```python
from build123d import *

# Parameters (mm, degrees)
SKETCH1_R           = 14
BOSS_EXTRUDE1_DEPTH = 10
SKETCH2_R           = 2.25
CUT_EXTRUDE1_DEPTH  = 5
SKETCH3_R           = 5
CUT_EXTRUDE2_DEPTH  = 1.8
SKETCH4_W           = 10
SKETCH4_H           = 10
BOSS_EXTRUDE2_DEPTH = 8
SKETCH6_W           = 8
SKETCH6_H           = 9.912865289
BOSS_EXTRUDE3_DEPTH = 20
CUT_EXTRUDE3_DEPTH  = 30
BOSS_EXTRUDE4_DEPTH = 80
SKETCH9_W           = 60
SKETCH9_H           = 60
CUT_EXTRUDE4_DEPTH  = 100


with BuildPart() as part:
    # Sketch1 → Boss-Extrude1 (new body)
    with BuildSketch(Plane.XY):
        Circle(SKETCH1_R)
    extrude(amount=BOSS_EXTRUDE1_DEPTH)

    # Sketch2 → Cut-Extrude1 (cut)
    with BuildSketch(Plane(origin=(0, 0, 0), x_dir=(-1, 0, 0), z_dir=(0, 0, -1))):
        Circle(SKETCH2_R)
    extrude(amount=-CUT_EXTRUDE1_DEPTH, mode=Mode.SUBTRACT)

    # Sketch3 → Cut-Extrude2 (cut)
    with BuildSketch(Plane(origin=(0, 0, 0), x_dir=(-1, 0, 0), z_dir=(0, 0, -1))):
        Circle(SKETCH3_R)
    extrude(amount=-CUT_EXTRUDE2_DEPTH, mode=Mode.SUBTRACT)

    # Sketch4 → Boss-Extrude2 (add)
    with BuildSketch(Plane.XY.offset(10)):
        Rectangle(SKETCH4_W, SKETCH4_H)
    extrude(amount=BOSS_EXTRUDE2_DEPTH)

    # Sketch6 → Boss-Extrude3 (add)
    with BuildSketch(Plane.ZY.offset(5)):
        with Locations((14, -0.043567356)):
            Rectangle(SKETCH6_W, SKETCH6_H)
    extrude(amount=BOSS_EXTRUDE3_DEPTH)

    # Sketch7 → Cut-Extrude3 (cut)
    with BuildSketch(Plane(origin=(5, 0, 0), x_dir=(0, 0, -1), z_dir=(1, 0, 0))):
        with BuildLine():
            Line((-18, 5), (-18, -5))
            Line((-18, -5), (-14, -5))
            ThreePointArc((-14, -5), (-14.330383596, 0), (-14, 5))
            Line((-14, 5), (-18, 5))
        make_face()
    extrude(amount=-CUT_EXTRUDE3_DEPTH, mode=Mode.SUBTRACT)

    # Sketch8 → Boss-Extrude4 (add)
    with BuildSketch(Plane.ZY.offset(25)):
        with BuildLine():
            Line((-62.16885098, 14.403585903), (13.83114902, 14.403585903))
            ThreePointArc((13.83114902, 14.403585903), (14.156322075, -2.818810644), (14, -20.043567356))
            Line((14, -20.043567356), (-62, -20.043567356))
            ThreePointArc((-62, -20.043567356), (-62.363996537, -2.821361111), (-62.16885098, 14.403585903))
        make_face()
    extrude(amount=BOSS_EXTRUDE4_DEPTH)

    # Sketch9 → Cut-Extrude4 (cut)
    with BuildSketch(Plane(origin=(0, 14.403585903, 0), x_dir=(1, 0, 0), z_dir=(0, 1, 0))):
        with Locations((-65, 24.16885098)):
            Rectangle(SKETCH9_W, SKETCH9_H)
    extrude(amount=-CUT_EXTRUDE4_DEPTH, mode=Mode.SUBTRACT)


solid = part.part
```
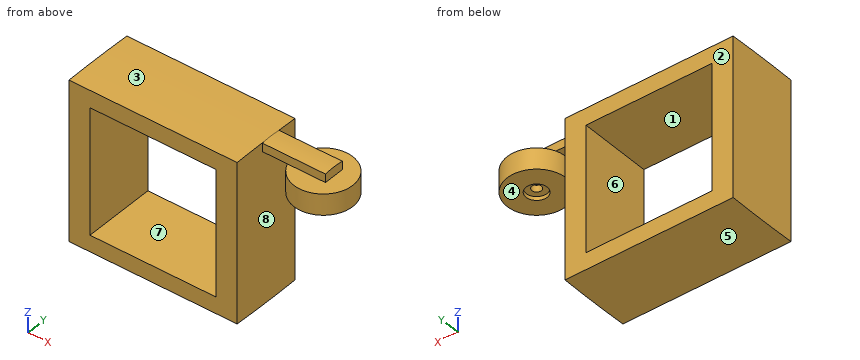
Geometry: final body of the model. Coordinates: model frame, mm. Face numbers are marked on the shaded views. A direction names the side the tool comes from. Coordinates: 2 decimals unless noted, no trailing zeros. Loops run counter-clockwise (first coordinate to the right, second up) from the corner with the lowest first, then second, coordinate; pieces in that order, holes last. Notation, with made-up numbers: (84.25, -22) -> (95.25, -22) arc R18 cw to (95.25, 6) -> close; hole circle Ø8 at (40, 79). An arc over 180 degrees is marked (long way). Use a Markdown table: item, result. Add a question column.
(1) Section query B-B, the plane z = -33.5. Return loops of the section in (x, y), plus the area to 3 significant figures.
(2) Mould query, pull axis Z, two halves, no side actions, for the marked faces 5, 6, 7 and 8. Classes: pulls with the +Z half, pulls with the -Z half, needs draft (parallel to the pull), parting line crosses it, or undercut.
(3) Line query: line 1 along X through (y, z) = (-0.5, -27); line 2 along Z through (x, y) = (-87, -3); line 3 along Y through (x, z) = (0, 2.6). Output: solid intervals per line, ascending.
(4) Section query A-A, the plane y = -10. Return loops of the section in (x, z).
(5) Section query D-D, the plane x = 0. Return loops of the section in (y, z).
(6) Pin query (flat end, axial travel): pin 1 Ø10 at (x, y) = (-46.5, -10.5) entering from +Z; pin 2 Ø13.5 at (x, y) = (4, 5.5) entering from +Z; pin 3 Ø5 at (x, y) = (-39, -4) entering from -Z. Return the tip coordinate at first contact, or that it passes through.
(7) Section query C-C, the plane x = -73. Return loops of the section in (y, z).
(8) Access query for the marked faces 1, 2, 3 and 4. Directions: +Z, -Z, +X, -X, +Y, -Y. A direction counts if a zero-diameter tool reaches every point of the face in a straight line with its end or side. Return the directions, or none.
Answer:
| question | item | result |
|---|---|---|
| 1 | outline | (-105, -20.04) -> (-95, -20.04) -> (-95, 14.4) -> (-105, 14.4) -> close; (-35, -20.04) -> (-25, -20.04) -> (-25, 14.4) -> (-35, 14.4) -> close |
| 1 | area | 689 mm^2 |
| 2 | face 5 | pulls with the -Z half |
| 2 | face 6 | undercut |
| 2 | face 7 | undercut |
| 2 | face 8 | needs draft |
| 3 | line 1 | x = -105 to -95, -35 to -25 |
| 3 | line 2 | z = -62.36 to -54.17, 5.83 to 14.16 |
| 3 | line 3 | y = -14 to -2.25, 2.25 to 14 |
| 4 | outline | (-105, -62.28) -> (-25, -62.28) -> (-25, 14.15) -> (-105, 14.15) -> close; (-9.8, 0) -> (9.8, 0) -> (9.8, 10) -> (-9.8, 10) -> close; hole (-95, -54.17) -> (-35, -54.17) -> (-35, 5.83) -> (-95, 5.83) -> close |
| 5 | outline | (-14, 0) -> (-5, 0) -> (-5, 1.8) -> (-2.25, 1.8) -> (-2.25, 5) -> (2.25, 5) -> (2.25, 1.8) -> (5, 1.8) -> (5, 0) -> (14, 0) -> (14, 10) -> (5, 10) -> (5, 14) arc R38 ccw to (-5, 14) -> (-5, 10) -> (-14, 10) -> close |
| 6 | pin 1 | stops at z = 14.16 |
| 6 | pin 2 | stops at z = 14.33 |
| 6 | pin 3 | stops at z = -62.37 |
| 7 | outline | (-20.04, -62) arc R530.69 ccw to (14.4, -62.17) -> (14.4, -54.17) -> (-20.04, -54.17) -> close; (-20.04, 5.83) -> (14.4, 5.83) -> (14.4, 13.83) arc R616.23 ccw to (-20.04, 14) -> close |
| 8 | face 1 | +Y, -Y |
| 8 | face 2 | +Z, -Z, +X, -X, +Y |
| 8 | face 3 | +Z, -X |
| 8 | face 4 | -Z, +X, +Y, -Y |
